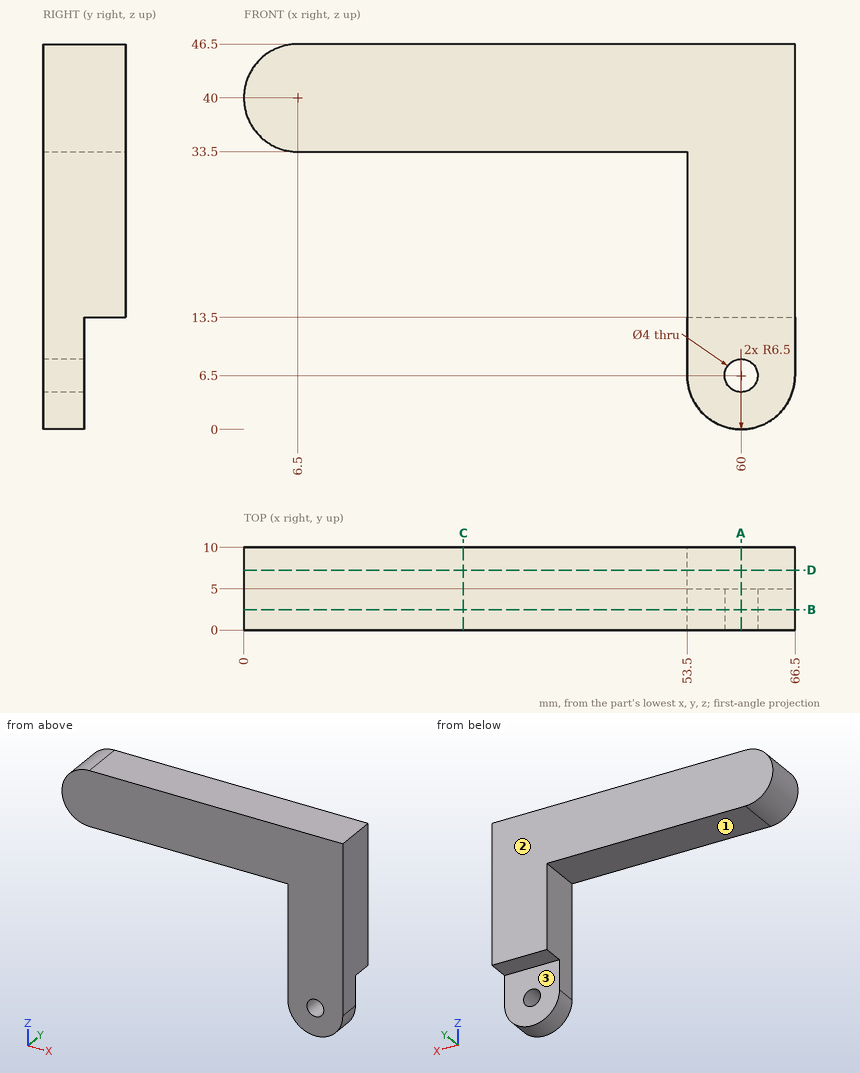
Study the drawing (mm; zero at the part's minimum x, y, z) and answer. A direction names the side the tool comes from. Round coordinates to 2 decimals unless told otherwise and drop trailing zeros. Loops run counter-clockwise (first coordinate to the right, second up) from the corner with the lowest first, then second, coordinate; pieces in that order, holes last.
Q1. Find the intervals of material crossed by line 1 (X direction, y = 1.9, z = 6.5); line 2 (X direction, y = 3.75, z = 16.5); line 3 (Z direction, x = 62, y = 6.25), in increasing order.
Q2. Section B-B, the plane y = 2.5 is taken. Determine the outline of the cut face in (x, z).
Q3. Given pin 1 Ø2 at (x, y) = (30.5, 1.5) entering from -Z; pin 2 Ø1.5 at (x, y) = (62, 7.5) entering from -Z; pin 3 Ø4 at (x, z) = (43.5, 39) entering from -Y; pin 4 Ø6.5 at (x, z) = (62, 9) entering from +Y, each flat-ended and moving along its own axis, determine where each tip first touches the part or whether it passes through.
Q4. Section C-C, the plane x = 26.5 is taken. Determine the outline of the cut face in (y, z), then the cut area to 3 significant figures.
Q5. Section D-D, the plane y = 7.25 is taken. Determine the outline of the cut face in (x, z), then the cut area to 3 significant figures.
Q6. Which of the six approach directions +Z, -Z, +X, -X, +Y, -Y give full straight-line access (tool end or side, diameter ignored) to the marked faces 1, 2 and 3?
Q7. Section A-A, the plane x = 60 is taken. Determine the outline of the cut face in (y, z).
Completed:
1. line 1: x = 53.5 to 58, 62 to 66.5
1. line 2: x = 53.5 to 66.5
1. line 3: z = 13.5 to 46.5
2. outline: (6.5, 33.5) - (53.5, 33.5) - (53.5, 6.5) arc R6.5 ccw to (66.5, 6.5) - (66.5, 46.5) - (6.5, 46.5) arc R6.5 ccw to start; hole circle Ø4 at (60, 6.5)
3. pin 1: stops at z = 33.5
3. pin 2: stops at z = 13.5
3. pin 3: stops at y = 0
3. pin 4: stops at y = 5
4. outline: (0, 33.5) - (10, 33.5) - (10, 46.5) - (0, 46.5) - close
4. area: 130 mm2
5. outline: (6.5, 33.5) - (53.5, 33.5) - (53.5, 13.5) - (66.5, 13.5) - (66.5, 46.5) - (6.5, 46.5) arc R6.5 ccw to start
5. area: 1,110 mm2
6. face 1: -Z, -X, +Y, -Y
6. face 2: +Z, -Z, +X, -X, +Y
6. face 3: -Z, +X, -X, +Y
7. outline: (0, 0) - (5, 0) - (5, 4.5) - (0, 4.5) - close; (0, 8.5) - (5, 8.5) - (5, 13.5) - (10, 13.5) - (10, 46.5) - (0, 46.5) - close
